Model file for the job. Use its own axes, mm. Face numbers are marked on the shaded views. A direction names the side the tool comes from. Coordinates: 2 decimals unless noted, no trailing zeros. Write each loop counter-clockwise with the first axis right and the second up, starting at its lowest first coordinate (ties: lowest second). Pieces come first, ordered by that corner, then holes. Notation, with made-up numbers: M -6,21.5 L -1,21.5 A30 cw -1,46.5 Z; hole C -35.75,19.5 d3. An arc over 180 degrees is marked long. Put each result on its own line as item: value. Start each with the question number.
Q1. Drill centre lines: line 1 along X through (y, z) = (6.25, -1.2); line 2 along Z through (x, y) = (1.55, 5.5); line 3 along Y through (x, z) = (2.3, -0.2). Where is each one in solid material? Low to high.
Q2. Which spindle directions (+Z, -Z, +X, -X, +Y, -Y) get a long thin tool onto all of the face, cutting with end or side? Do the marked faces 1, 2 and 3. Say none if no direction does.
Q3. Cut at A-A (z = -1.4). Write the cut outline in (x, y), then the cut area to 3 significant figures.
Q4. Cut at C-C (x = 0.25). Write the cut outline in (y, z), then the cut area to 3 significant figures.
Q5. Cut at B-B (y = 3.25). Write the cut outline in (x, z), then the cut area to 3 significant figures.
Q6. Cut at D-D (z = -2.1). Write the cut outline in (x, y).
Q7. Pull direction X, two halves, no side cores. Call the marked faces 4, 5, 6 and 7: pulls with the +X half, pulls with the -X half, needs draft (parallel to the pull), parting line crosses it, or undercut.
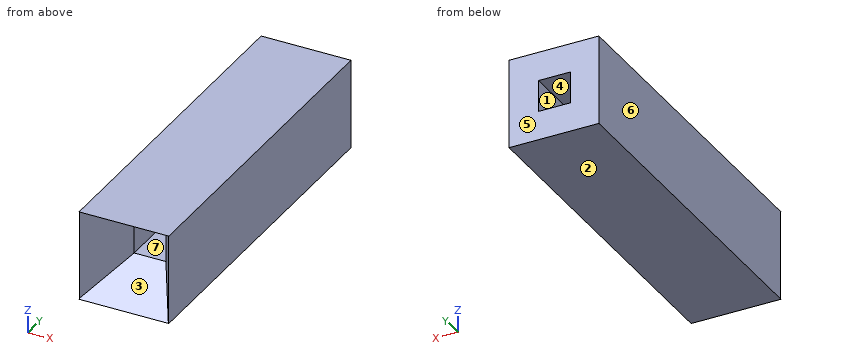
```python
from build123d import *

# Parameters (mm, degrees)
SKETCH1_W           = 2.83333
SKETCH1_H           = 2.83333
BOSS_EXTRUDE2_DEPTH = 11
SKETCH2_W           = 1
SKETCH2_H           = 1
CUT_EXTRUDE1_DEPTH  = 11


with BuildPart() as part:
    # Sketch1 → Boss-Extrude2 (new body)
    with BuildSketch(Plane(origin=(0, 0, 0), x_dir=(1, 0, 0), z_dir=(0, 1, 0))):
        with Locations((1.416665, 1.416665)):
            Rectangle(SKETCH1_W, SKETCH1_H)
    extrude(amount=BOSS_EXTRUDE2_DEPTH)

    # Sketch2 → Cut-Extrude1 (cut)
    with BuildSketch(Plane(origin=(0, 0, 0), x_dir=(-1, 0, 0), z_dir=(0, -1, 0))):
        with Locations((-1.4, 1.416665)):
            Rectangle(SKETCH2_W, SKETCH2_H)
    extrude(amount=-CUT_EXTRUDE1_DEPTH, mode=Mode.SUBTRACT)

    # Chamfer5
    # the kernel refuses this chamfer: 1.732050808, 1 mm, written as the material it takes off along each edge
    with BuildSketch(Plane(origin=(1.9, 0, -0.916665), x_dir=(0, -0.05789386240267139, 0.9983227437537926), z_dir=(-1, 0, 0)), Plane(origin=(0.9, 0, -0.916665), x_dir=(-0.9983227437537926, -0.0578938624026714, 0), z_dir=(0, 0, -1)), Plane(origin=(0.9, 0, -1.916665), x_dir=(0, -0.05789386240267139, -0.9983227437537926), z_dir=(1, 0, 0)), Plane(origin=(1.9, 0, -1.916665), x_dir=(0.9983227437537926, -0.05789386240267139, 0), z_dir=(0, 0, 1))) as chamfer5_piece_1:
        with BuildLine():
            Line((1.03637929, 0), (-0.138331657, 1.787039577))
            Line((-0.138331657, 1.787039577), (-0.172914571, 1.785034075))
            ThreePointArc((-0.172914571, 1.785034075), (-0.086457286, 0.892517037), (-0.034582914, -0.002005502))
            Line((-0.034582914, -0.002005502), (0.002005502, -0.034582914))
            ThreePointArc((0.002005502, -0.034582914), (0.518458331, -0.004633232), (1.038384792, -0.034582914))
            Line((1.038384792, -0.034582914), (1.03637929, 0))
        make_face()
    extrude(amount=1, mode=Mode.SUBTRACT)
    with BuildSketch(Plane(origin=(1.9, 0, -1.916665), x_dir=(0.9983227437537926, -0.05789386240267139, 0), z_dir=(0, 0, 1))) as chamfer5_piece_2a_section:
        with BuildLine():
            Line((1.03637929, 0), (-0.138331657, 1.787039577))
            Line((-0.138331657, 1.787039577), (-0.172914571, 1.785034075))
            ThreePointArc((-0.172914571, 1.785034075), (-0.086457286, 0.892517037), (-0.034582914, -0.002005502))
            Line((-0.034582914, -0.002005502), (0.002005502, -0.034582914))
            ThreePointArc((0.002005502, -0.034582914), (0.518458331, -0.004633232), (1.038384792, -0.034582914))
            Line((1.038384792, -0.034582914), (1.03637929, 0))
        make_face()
    chamfer5_piece_2a = extrude(amount=5.480963971, mode=Mode.PRIVATE)
    chamfer5_piece_2a = split(chamfer5_piece_2a, bisect_by=Plane(origin=(2.220669895, 0.580899134, -0.916665), z_dir=(0, 0, 1)), keep=Keep.TOP, mode=Mode.PRIVATE)
    with BuildSketch(Plane(origin=(6.380963971, 0, -0.916665), x_dir=(0, -0.05789386240267139, 0.9983227437537926), z_dir=(-1, 0, 0))) as chamfer5_piece_2b_section:
        with BuildLine():
            Line((1.03637929, 0), (-0.138331657, 1.787039577))
            Line((-0.138331657, 1.787039577), (-0.172914571, 1.785034075))
            ThreePointArc((-0.172914571, 1.785034075), (-0.086457286, 0.892517037), (-0.034582914, -0.002005502))
            Line((-0.034582914, -0.002005502), (0.002005502, -0.034582914))
            ThreePointArc((0.002005502, -0.034582914), (0.518458331, -0.004633232), (1.038384792, -0.034582914))
            Line((1.038384792, -0.034582914), (1.03637929, 0))
        make_face()
    chamfer5_piece_2b = extrude(amount=5.480963971, mode=Mode.PRIVATE)
    chamfer5_piece_2b = split(chamfer5_piece_2b, bisect_by=Plane(origin=(1.9, 0.580899134, -0.595995105), z_dir=(1, 0, 0)), keep=Keep.TOP, mode=Mode.PRIVATE)
    chamfer5_piece_2 = chamfer5_piece_2a & chamfer5_piece_2b
    add(chamfer5_piece_2, mode=Mode.SUBTRACT)
    with BuildSketch(Plane(origin=(0.9, 0, 3.564298971), x_dir=(-0.9983227437537926, -0.0578938624026714, 0), z_dir=(0, 0, -1))) as chamfer5_piece_3a_section:
        with BuildLine():
            Line((1.03637929, 0), (-0.138331657, 1.787039577))
            Line((-0.138331657, 1.787039577), (-0.172914571, 1.785034075))
            ThreePointArc((-0.172914571, 1.785034075), (-0.086457286, 0.892517037), (-0.034582914, -0.002005502))
            Line((-0.034582914, -0.002005502), (0.002005502, -0.034582914))
            ThreePointArc((0.002005502, -0.034582914), (0.518458331, -0.004633232), (1.038384792, -0.034582914))
            Line((1.038384792, -0.034582914), (1.03637929, 0))
        make_face()
    chamfer5_piece_3a = extrude(amount=5.480963971, mode=Mode.PRIVATE)
    chamfer5_piece_3a = split(chamfer5_piece_3a, bisect_by=Plane(origin=(0.579330105, 0.580899134, -0.916665), z_dir=(0, 0, 1)), keep=Keep.TOP, mode=Mode.PRIVATE)
    with BuildSketch(Plane(origin=(1.9, 0, -0.916665), x_dir=(0, -0.05789386240267139, 0.9983227437537926), z_dir=(-1, 0, 0))) as chamfer5_piece_3b_section:
        with BuildLine():
            Line((1.03637929, 0), (-0.138331657, 1.787039577))
            Line((-0.138331657, 1.787039577), (-0.172914571, 1.785034075))
            ThreePointArc((-0.172914571, 1.785034075), (-0.086457286, 0.892517037), (-0.034582914, -0.002005502))
            Line((-0.034582914, -0.002005502), (0.002005502, -0.034582914))
            ThreePointArc((0.002005502, -0.034582914), (0.518458331, -0.004633232), (1.038384792, -0.034582914))
            Line((1.038384792, -0.034582914), (1.03637929, 0))
        make_face()
    chamfer5_piece_3b = extrude(amount=5.480963971, mode=Mode.PRIVATE)
    chamfer5_piece_3b = split(chamfer5_piece_3b, bisect_by=Plane(origin=(0.9, 0.580899134, -0.595995105), z_dir=(-1, 0, 0)), keep=Keep.TOP, mode=Mode.PRIVATE)
    chamfer5_piece_3 = chamfer5_piece_3a & chamfer5_piece_3b
    add(chamfer5_piece_3, mode=Mode.SUBTRACT)
    with BuildSketch(Plane(origin=(-3.580963971, 0, -1.916665), x_dir=(0, -0.05789386240267139, -0.9983227437537926), z_dir=(1, 0, 0))) as chamfer5_piece_4a_section:
        with BuildLine():
            Line((1.03637929, 0), (-0.138331657, 1.787039577))
            Line((-0.138331657, 1.787039577), (-0.172914571, 1.785034075))
            ThreePointArc((-0.172914571, 1.785034075), (-0.086457286, 0.892517037), (-0.034582914, -0.002005502))
            Line((-0.034582914, -0.002005502), (0.002005502, -0.034582914))
            ThreePointArc((0.002005502, -0.034582914), (0.518458331, -0.004633232), (1.038384792, -0.034582914))
            Line((1.038384792, -0.034582914), (1.03637929, 0))
        make_face()
    chamfer5_piece_4a = extrude(amount=5.480963971, mode=Mode.PRIVATE)
    chamfer5_piece_4a = split(chamfer5_piece_4a, bisect_by=Plane(origin=(0.9, 0.580899134, -2.237334895), z_dir=(-1, 0, 0)), keep=Keep.TOP, mode=Mode.PRIVATE)
    with BuildSketch(Plane(origin=(0.9, 0, -0.916665), x_dir=(-0.9983227437537926, -0.0578938624026714, 0), z_dir=(0, 0, -1))) as chamfer5_piece_4b_section:
        with BuildLine():
            Line((1.03637929, 0), (-0.138331657, 1.787039577))
            Line((-0.138331657, 1.787039577), (-0.172914571, 1.785034075))
            ThreePointArc((-0.172914571, 1.785034075), (-0.086457286, 0.892517037), (-0.034582914, -0.002005502))
            Line((-0.034582914, -0.002005502), (0.002005502, -0.034582914))
            ThreePointArc((0.002005502, -0.034582914), (0.518458331, -0.004633232), (1.038384792, -0.034582914))
            Line((1.038384792, -0.034582914), (1.03637929, 0))
        make_face()
    chamfer5_piece_4b = extrude(amount=5.480963971, mode=Mode.PRIVATE)
    chamfer5_piece_4b = split(chamfer5_piece_4b, bisect_by=Plane(origin=(0.579330105, 0.580899134, -1.916665), z_dir=(0, 0, -1)), keep=Keep.TOP, mode=Mode.PRIVATE)
    chamfer5_piece_4 = chamfer5_piece_4a & chamfer5_piece_4b
    add(chamfer5_piece_4, mode=Mode.SUBTRACT)
    with BuildSketch(Plane(origin=(1.9, 0, -6.397628971), x_dir=(0.9983227437537926, -0.05789386240267139, 0), z_dir=(0, 0, 1))) as chamfer5_piece_5a_section:
        with BuildLine():
            Line((1.03637929, 0), (-0.138331657, 1.787039577))
            Line((-0.138331657, 1.787039577), (-0.172914571, 1.785034075))
            ThreePointArc((-0.172914571, 1.785034075), (-0.086457286, 0.892517037), (-0.034582914, -0.002005502))
            Line((-0.034582914, -0.002005502), (0.002005502, -0.034582914))
            ThreePointArc((0.002005502, -0.034582914), (0.518458331, -0.004633232), (1.038384792, -0.034582914))
            Line((1.038384792, -0.034582914), (1.03637929, 0))
        make_face()
    chamfer5_piece_5a = extrude(amount=5.480963971, mode=Mode.PRIVATE)
    chamfer5_piece_5a = split(chamfer5_piece_5a, bisect_by=Plane(origin=(2.220669895, 0.580899134, -1.916665), z_dir=(0, 0, -1)), keep=Keep.TOP, mode=Mode.PRIVATE)
    with BuildSketch(Plane(origin=(0.9, 0, -1.916665), x_dir=(0, -0.05789386240267139, -0.9983227437537926), z_dir=(1, 0, 0))) as chamfer5_piece_5b_section:
        with BuildLine():
            Line((1.03637929, 0), (-0.138331657, 1.787039577))
            Line((-0.138331657, 1.787039577), (-0.172914571, 1.785034075))
            ThreePointArc((-0.172914571, 1.785034075), (-0.086457286, 0.892517037), (-0.034582914, -0.002005502))
            Line((-0.034582914, -0.002005502), (0.002005502, -0.034582914))
            ThreePointArc((0.002005502, -0.034582914), (0.518458331, -0.004633232), (1.038384792, -0.034582914))
            Line((1.038384792, -0.034582914), (1.03637929, 0))
        make_face()
    chamfer5_piece_5b = extrude(amount=5.480963971, mode=Mode.PRIVATE)
    chamfer5_piece_5b = split(chamfer5_piece_5b, bisect_by=Plane(origin=(1.9, 0.580899134, -2.237334895), z_dir=(1, 0, 0)), keep=Keep.TOP, mode=Mode.PRIVATE)
    chamfer5_piece_5 = chamfer5_piece_5a & chamfer5_piece_5b
    add(chamfer5_piece_5, mode=Mode.SUBTRACT)


solid = part.part
```
Computed values:
1. line 1: 0 to 0.9, 1.9 to 2.83
1. line 2: -2.83 to -1.92, -0.92 to 0
1. line 3: 0.49 to 11
2. face 1: +Y, -Y
2. face 2: -Z, +X, -X, +Y, -Y
2. face 3: -Y
3. outline: M 0,0.17 L 0.9,1.73 L 0.9,11 L 0,11 Z; M 1.9,1.73 L 2.83,0.12 L 2.83,11 L 1.9,11 Z
3. area: 18.4 mm2
4. outline: M 0.14,-2.83 L 11,-2.83 L 11,0 L 0.14,0 L 0.61,-0.27 L 0.61,-2.57 Z
4. area: 29.6 mm2
5. outline: M 0,-2.83 L 2.83,-2.83 L 2.83,0 L 0,0 Z; hole M 0.9,-1.92 L 1.9,-1.92 L 1.9,-0.92 L 0.9,-0.92 Z
5. area: 7.03 mm2
6. outline: M 0,0.17 L 0.72,1.41 L 2.08,1.41 L 2.83,0.12 L 2.83,11 L 0,11 Z
7. face 4: undercut
7. face 5: needs draft
7. face 6: pulls with the -X half
7. face 7: undercut
